Autodesk Inventor part; units mm, degrees
ref_plane "YZ Plane" through (0, 0, 0) normal (1, 0, 0) x (0, 1, 0)
ref_plane "XZ Plane" through (0, 0, 0) normal (0, 1, 0) x (-1, 0, 0)
ref_plane "XY Plane" through (0, 0, 0) normal (0, 0, 1) x (1, 0, 0)
sketch "Base" plane through (0, 0, 0) normal (0, 0, 1) x (1, 0, 0)
  circle A0 centre (0, 0) radius 16
  circle A1 centre (0, 0) radius 7
  circle A2 centre (0, 0) radius 11.3137 construction
  line L0 (-8, 8) -> (8, 8) construction
  line L1 (8, 8) -> (8, -8) construction
  line L2 (8, -8) -> (-8, -8) construction
  line L3 (-8, -8) -> (-8, 8) construction
  circle A3 centre (-8, 8) radius 2
  circle A4 centre (8, 8) radius 2
  circle A5 centre (-8, -8) radius 2
  circle A6 centre (8, -8) radius 2
  circle A7 centre (-11.3137, 0) radius 2
  circle A8 centre (0, 11.3137) radius 2
  line L4 (0, 8) -> (0, -8) construction
  circle A9 centre (11.3137, 0) radius 2
  line L5 (-8, 0) -> (8, 0) construction
  line L6 (0, 11.3137) -> (0, 0) construction
  line L7 (0, 11.3137) -> (0, -8) construction
  line L8 (-11.3137, 0) -> (0, 0) construction
  circle A10 centre (0, -11.3137) radius 2
  line L9 (0, -11.3137) -> (0, 0) construction
  dimension "d0" = 32
  dimension "d1" = 14
  dimension "d2" = 4
  dimension "d3" = 4
  dimension "d4" = 4
  dimension "d5" = 4
  dimension "d6" = 16
extrude "BaseFeature" add sketch "Base" along normal blind 6
sketch "Indent" plane through (0, 0, 6) normal (0, 0, 1) x (1, 0, 0)
  circle A0 centre (0, 0) radius 8
  dimension "d9" = 16
extrude "IndentFeature" cut sketch "Indent" against normal blind 1
sketch "ShoulderJointPoint" plane through (0, 0, 6) normal (0, 0, 1) x (1, 0, 0)
  point P0 (0, 0)
properties part number "PatternSpacer4mm" material "Aluminum 6061"
Build history of the part. All positions in model axes, mm. A direction names the side the tool comes from. Round coordinates to 2 decimals unless told otherwise and drop trailing zeros. Write each loop counter-clockwise with the first axis right and the second up, starting at its lowest first coordinate (ties: lowest second). Pieces come first, ordered by that corner, then holes.
1) 3-axis set-ups, long thin cutter, end or side, ignore diameter. For faces 1 (the cylindrical face through (6, 8, 3)), 2 (the flat face through (4, -6, 5)): which of +Z, -Z, +X, -X, +Y, -Y reach the whole face in a straight line?
2) Band-saw the part on B-B, the plane x = -12. List the corners of the cut face in (y, z), and give its area (3 significant figures).
3) Drill centre lines: probe 1 along Y at (x, z) = (0, 5.4); probe 2 along Y at (x, z) = (-0.5, 4.5); probe 3 along X at (y, z) = (9, 1). Where is each one in solid material? Low to high.
4) Band-saw the part on C-C, the plane z = 5.55. Give the number of separate pieces and of enclosed holes in the cut face, and give its area (3 significant figures).
5) Pin check, flat tips, straight feed: pin 1 (3.5 mm diameter, centred on x = 8, y = -8, fed in from -Z); pin 2 (5 mm diameter, centred on x = -8, y = -8, fed in from -Z); pin 3 (1 mm diameter, centred on y = -9, z = 4.5, fed in from +X); pin 4 (1.5 mm diameter, centred on y = 2, z = 4, fed in from -X). Stop position of each tip, or through.
6) Band-saw the part on A-A, the plane y = 0. List the corners of the cut face in (x, z), and give its area (3 significant figures).
Ans:
1. face 1: +Z, -Z
1. face 2: +Z
2. outline: (-10.58, 0) - (-1.88, 0) - (-1.88, 6) - (-10.58, 6) - close; (1.88, 0) - (10.58, 0) - (10.58, 6) - (1.88, 6) - close
2. area: 104 mm2
3. probe 1: y = -16 to -13.31, -9.31 to -8, 8 to 9.31, 13.31 to 16
3. probe 2: y = -15.99 to -13.25, -9.38 to -6.98, 6.98 to 9.38, 13.25 to 15.99
3. probe 3: x = -13.23 to -9.73, -6.27 to 6.27, 9.73 to 13.23
4. separate pieces: 1
4. enclosed holes: 9
4. area: 503 mm2
5. pin 1: passes through
5. pin 2: stops at z = 0
5. pin 3: stops at x = 13.56
5. pin 4: stops at x = -15.95
6. outline: (-16, 0) - (-13.31, 0) - (-13.31, 6) - (-16, 6) - close; (-9.31, 0) - (-7, 0) - (-7, 5) - (-8, 5) - (-8, 6) - (-9.31, 6) - close; (7, 0) - (9.31, 0) - (9.31, 6) - (8, 6) - (8, 5) - (7, 5) - close; (13.31, 0) - (16, 0) - (16, 6) - (13.31, 6) - close
6. area: 58.0 mm2
